Geometry check sheet. Reference: the model listing, model coordinates, mm. Round coordinates to 2 decimals unless told otherwise and drop trailing zeros. Write each loop counter-clockwise with the first axis right and the second up, starting at its lowest first coordinate (ties: lowest second). Pieces come first, ordered by that corner, then holes. Notation, with made-up numbers: (36.5, 33) -> (71.5, 33) arc R15 ccw to (71.5, 52) -> close; hole circle Ø1 at (-23, 47). An arc over 180 degrees is marked (long way). Use a Markdown table: item, result.
```python
from build123d import *

# Parameters (mm, degrees)
SKETCH4_R           = 39
BOSS_EXTRUDE1_DEPTH = 3
CUT_EXTRUDE1_DEPTH  = 3
SKETCH1_R           = 6.096
SKETCH1_R_2         = 1.7859375
CUT_EXTRUDE3_DEPTH  = 3
FILLET1_R           = 1


with BuildPart() as part:
    # Sketch4 → Boss-Extrude1 (new body)
    with BuildSketch(Plane(origin=(0, 0, 0), x_dir=(1, 0, 0), z_dir=(0, 1, 0))):
        Circle(SKETCH4_R)
    extrude(amount=BOSS_EXTRUDE1_DEPTH)

    # Sketch3 → Cut-Extrude1 (cut)
    with BuildSketch(Plane(origin=(0, 0, 0), x_dir=(1, 0, 0), z_dir=(0, 1, 0))):
        with BuildLine():
            Line((32.968591312, 1.439439783), (35.965735977, 1.570297945))
            ThreePointArc((35.965735977, 1.570297945), (34.561794758, 10.073844505), (31.176914536, 18))
            Line((31.176914536, 18), (28.578838325, 16.5))
            ThreePointArc((28.578838325, 16.5), (31.681645195, 9.234357463), (32.968591312, 1.439439783))
        make_face()
        with BuildLine():
            Line((-1.570297945, 35.965735977), (-1.439439783, 32.968591312))
            ThreePointArc((-1.439439783, 32.968591312), (2.158303265, 32.929344467), (5.730389863, 32.498655849))
            Line((5.730389863, 32.498655849), (6.186823022, 35.464393705))
            ThreePointArc((6.186823022, 35.464393705), (2.321833751, 35.925048198), (-1.570297945, 35.965735977))
        make_face()
        with BuildLine():
            Line((12.31272516, 33.828934348), (11.28666473, 31.009856486))
            ThreePointArc((11.28666473, 31.009856486), (13.946402637, 29.908156972), (16.5, 28.578838325))
            Line((16.5, 28.578838325), (18, 31.176914536))
            ThreePointArc((18, 31.176914536), (15.214257423, 32.627080333), (12.31272516, 33.828934348))
        make_face()
        with BuildLine():
            Line((23.163459499, 27.558195587), (21.21199112, 25.279466623))
            ThreePointArc((21.21199112, 25.279466623), (23.334523779, 23.334523779), (25.279466623, 21.21199112))
            Line((25.279466623, 21.21199112), (27.577599952, 23.140353949))
            ThreePointArc((27.577599952, 23.140353949), (25.466509571, 25.445174203), (23.163459499, 27.558195587))
        make_face()
        with BuildLine():
            Line((14.985723324, -0.65429081), (17.982867988, -0.785148973))
            ThreePointArc((17.982867988, -0.785148973), (16.143709348, 7.961196424), (10.324375854, 14.744736797))
            Line((10.324375854, 14.744736797), (8.603646545, 12.287280664))
            ThreePointArc((8.603646545, 12.287280664), (13.453091123, 6.634330353), (14.985723324, -0.65429081))
        make_face()
        with BuildLine():
            Line((2.614672282, 29.885840943), (2.353205054, 26.897256848))
            ThreePointArc((2.353205054, 26.897256848), (6.988114218, 26.07999731), (11.410693067, 24.47031025))
            Line((11.410693067, 24.47031025), (12.678547852, 27.189233611))
            ThreePointArc((12.678547852, 27.189233611), (7.764571353, 28.977774789), (2.614672282, 29.885840943))
        make_face()
        with BuildLine():
            Line((21.213203436, 21.213203436), (19.091883092, 19.091883092))
            ThreePointArc((19.091883092, 19.091883092), (22.117105196, 15.486563781), (24.47031025, 11.410693067))
            Line((24.47031025, 11.410693067), (27.189233611, 12.678547852))
            ThreePointArc((27.189233611, 12.678547852), (24.574561329, 17.207293091), (21.213203436, 21.213203436))
        make_face()
        with BuildLine():
            Line((6.211657082, 23.182219831), (5.435199947, 20.284442352))
            ThreePointArc((5.435199947, 20.284442352), (12.045105163, 17.20219293), (17.20219293, 12.045105163))
            Line((17.20219293, 12.045105163), (19.659649063, 13.765834472))
            ThreePointArc((19.659649063, 13.765834472), (13.765834472, 19.659649063), (6.211657082, 23.182219831))
        make_face()
        with BuildLine():
            Line((-32.968591312, -1.439439783), (-35.965735977, -1.570297945))
            ThreePointArc((-35.965735977, -1.570297945), (-34.561794758, -10.073844505), (-31.176914536, -18))
            Line((-31.176914536, -18), (-28.578838325, -16.5))
            ThreePointArc((-28.578838325, -16.5), (-31.681645195, -9.234357463), (-32.968591312, -1.439439783))
        make_face()
        with BuildLine():
            Line((1.570297945, -35.965735977), (1.439439783, -32.968591312))
            ThreePointArc((1.439439783, -32.968591312), (-2.158303265, -32.929344467), (-5.730389863, -32.498655849))
            Line((-5.730389863, -32.498655849), (-6.186823022, -35.464393705))
            ThreePointArc((-6.186823022, -35.464393705), (-2.321833751, -35.925048198), (1.570297945, -35.965735977))
        make_face()
        with BuildLine():
            Line((-12.31272516, -33.828934348), (-11.28666473, -31.009856486))
            ThreePointArc((-11.28666473, -31.009856486), (-13.946402637, -29.908156972), (-16.5, -28.578838325))
            Line((-16.5, -28.578838325), (-18, -31.176914536))
            ThreePointArc((-18, -31.176914536), (-15.214257423, -32.627080333), (-12.31272516, -33.828934348))
        make_face()
        with BuildLine():
            Line((-23.163459499, -27.558195587), (-21.21199112, -25.279466623))
            ThreePointArc((-21.21199112, -25.279466623), (-23.334523779, -23.334523779), (-25.279466623, -21.21199112))
            Line((-25.279466623, -21.21199112), (-27.577599952, -23.140353949))
            ThreePointArc((-27.577599952, -23.140353949), (-25.466509571, -25.445174203), (-23.163459499, -27.558195587))
        make_face()
        with BuildLine():
            Line((-14.985723324, 0.65429081), (-17.982867988, 0.785148973))
            ThreePointArc((-17.982867988, 0.785148973), (-16.143709348, -7.961196424), (-10.324375854, -14.744736797))
            Line((-10.324375854, -14.744736797), (-8.603646545, -12.287280664))
            ThreePointArc((-8.603646545, -12.287280664), (-13.453091123, -6.634330353), (-14.985723324, 0.65429081))
        make_face()
        with BuildLine():
            Line((-2.614672282, -29.885840943), (-2.353205054, -26.897256848))
            ThreePointArc((-2.353205054, -26.897256848), (-6.988114218, -26.07999731), (-11.410693067, -24.47031025))
            Line((-11.410693067, -24.47031025), (-12.678547852, -27.189233611))
            ThreePointArc((-12.678547852, -27.189233611), (-7.764571353, -28.977774789), (-2.614672282, -29.885840943))
        make_face()
        with BuildLine():
            Line((-21.213203436, -21.213203436), (-19.091883092, -19.091883092))
            ThreePointArc((-19.091883092, -19.091883092), (-22.117105196, -15.486563781), (-24.47031025, -11.410693067))
            Line((-24.47031025, -11.410693067), (-27.189233611, -12.678547852))
            ThreePointArc((-27.189233611, -12.678547852), (-24.574561329, -17.207293091), (-21.213203436, -21.213203436))
        make_face()
        with BuildLine():
            Line((-6.211657082, -23.182219831), (-5.435199947, -20.284442352))
            ThreePointArc((-5.435199947, -20.284442352), (-12.045105163, -17.20219293), (-17.20219293, -12.045105163))
            Line((-17.20219293, -12.045105163), (-19.659649063, -13.765834472))
            ThreePointArc((-19.659649063, -13.765834472), (-13.765834472, -19.659649063), (-6.211657082, -23.182219831))
        make_face()
    extrude(amount=CUT_EXTRUDE1_DEPTH, mode=Mode.SUBTRACT)

    # Sketch1 → Cut-Extrude3 (cut)
    with BuildSketch(Plane(origin=(0, 0, 0), x_dir=(1, 0, 0), z_dir=(0, 1, 0))):
        Circle(SKETCH1_R)
        with Locations((6.914797213, 6.914797213)):
            Circle(SKETCH1_R_2)
        with Locations((6.914797213, -6.914797213)):
            Circle(SKETCH1_R_2)
        with Locations((-6.914797213, -6.914797213)):
            Circle(SKETCH1_R_2)
        with Locations((-6.914797213, 6.914797213)):
            Circle(SKETCH1_R_2)
    extrude(amount=CUT_EXTRUDE3_DEPTH, mode=Mode.SUBTRACT)

    # Fillet1
    fillet1_edges = [part.edges().sort_by_distance(p)[0] for p in [
        (-39, 0, 0),
        (-6.096, 0, 0),
        (-6.096, 3, 0),
        (-39, 3, 0),
    ]]
    fillet(fillet1_edges, radius=FILLET1_R)


solid = part.part
```
(1) Section check A-A on x = 0. Record the cut outline in (y, z).
A:
| item | result |
|---|---|
| outline | (0, -38) arc R1 ccw to (1, -39) -> (2, -39) arc R1 ccw to (3, -38) -> (3, -36) -> (0, -36) -> close; (0, -33) -> (3, -33) -> (3, -7.1) arc R1 ccw to (2, -6.1) -> (1, -6.1) arc R1 ccw to (0, -7.1) -> close; (0, 7.1) arc R1 ccw to (1, 6.1) -> (2, 6.1) arc R1 ccw to (3, 7.1) -> (3, 33) -> (0, 33) -> close; (0, 36) -> (3, 36) -> (3, 38) arc R1 ccw to (2, 39) -> (1, 39) arc R1 ccw to (0, 38) -> close |
(2) Gauge pin test, flat ends, axial feed: pin 1 Ø1 at (x, y) = (5.5, 1.5) entering from +Z; pin 2 Ø1 at (y, z) = (0.5, 4) entering from +X; pin 3 Ø6 at (x, z) = (-14, 0.5) entering from -Y. Record the tip position at first contact, or that the pin passes through.
A:
| item | result |
|---|---|
| pin 1 | stops at z = 38.68 |
| pin 2 | stops at x = 38.82 |
| pin 3 | stops at y = 0 |
(3) Thickness scan on line 1 (Z direction, x = 0, y = 1.7); line 2 (X direction, y = 2.2, z = 10.5); line 3 (Z direction, x = -26, y = 0.7). Record the ranges inside material, lowest first.
A:
| item | result |
|---|---|
| line 1 | z = -39 to -36, -33 to -6.1, 6.1 to 33, 36 to 39 |
| line 2 | x = -37.54 to -34.43, -31.28 to -14.62, -10.71 to 37.54 |
| line 3 | z = -29.01 to 12.12, 14.97 to 21.82, 24.9 to 29.01 |
